from build123d import *

# Parameters (mm, degrees)
RESSALTO_EXTRUS_O1_DEPTH = 500
CANAL_DEPTH              = 800
ESBO_O2_5_R              = 2.1
FURO_DEPTH               = 501.49975025
CORTE_EXTRUS_O4_DEPTH    = 501.49975025
PADR_OCIRCULAR2_COUNT    = 3
PADR_OCIRCULAR2_ANGLE    = 180
ESPELHAR2_COPY_1_DEPTH   = 800
ESPELHAR2_COPY_2_DEPTH   = 800


with BuildPart() as part:
    # Esboço1 → Ressalto-extrusão1 (new body)
    with BuildSketch(Plane.XY):
        with BuildLine():
            Line((-19, 10), (19, 10))
            ThreePointArc((19, 10), (19.707106781, 9.707106781), (20, 9))
            Line((20, 9), (20, -9))
            ThreePointArc((20, -9), (19.707106781, -9.707106781), (19, -10))
            Line((19, -10), (-19, -10))
            ThreePointArc((-19, -10), (-19.707106781, -9.707106781), (-20, -9))
            Line((-20, -9), (-20, 9))
            ThreePointArc((-20, 9), (-19.707106781, 9.707106781), (-19, 10))
        make_face()
    extrude(amount=RESSALTO_EXTRUS_O1_DEPTH)

    # Esboço2 → CANAL (cut)
    with BuildSketch(Plane.XY.offset(500)):
        Polygon((-14.8, 10), (-13, 8.2), (-15.5, 8.2), (-15.5, 6.560660172), (-12.939339828, 4), (-10.3, 4), (-10, 3.7), (-9.7, 4), (-7.060660172, 4), (-4.5, 6.560660172), (-4.5, 8.2), (-7, 8.2), (-5.2, 10), align=None)
    canal = extrude(amount=-CANAL_DEPTH, mode=Mode.SUBTRACT)

    # Esboço2<5> → FURO (cut, through all)
    with BuildSketch(Plane.XY.offset(500)):
        with Locations((-10, 0)):
            Circle(ESBO_O2_5_R)
    furo = extrude(amount=-FURO_DEPTH, mode=Mode.SUBTRACT)

    # Esboço2<6> → Corte-extrusão4 (cut, through all)
    with BuildSketch(Plane.XY.offset(500)):
        Polygon((-2.7, 8.2), (-2.7, 6.239339828), (-6, 2.939339828), (-6, 0), (6, 0), (6, 2.939339828), (2.7, 6.239339828), (2.7, 8.2), align=None)
    corte_extrus_o4 = extrude(amount=-CORTE_EXTRUS_O4_DEPTH, mode=Mode.SUBTRACT)

    # PadrãoCircular2: CANAL ×3 about axis
    padr_ocircular2_axis = Axis((-10, 0, 0), (0, 0, 1))
    for i in range(1, PADR_OCIRCULAR2_COUNT):
        add(canal.rotate(padr_ocircular2_axis, i * PADR_OCIRCULAR2_ANGLE / (PADR_OCIRCULAR2_COUNT - 1)), mode=Mode.SUBTRACT)

    # Espelhar2: CANAL, FURO, Corte-extrusão4 across plane
    add(canal.mirror(Plane(origin=(0, 0, 0), x_dir=(0, 0, 1), z_dir=(1, 0, 0))), mode=Mode.SUBTRACT)
    add(furo.mirror(Plane(origin=(0, 0, 0), x_dir=(0, 0, 1), z_dir=(1, 0, 0))), mode=Mode.SUBTRACT)
    add(corte_extrus_o4.mirror(Plane(origin=(0, 0, 0), x_dir=(0, 0, 1), z_dir=(1, 0, 0))), mode=Mode.SUBTRACT)

    # Espelhar2 copy 1 sketch → Espelhar2 copy 1 (cut)
    with BuildSketch(Plane(origin=(10, 10, 500), x_dir=(0, 1, 0), z_dir=(0, 0, 1))):
        Polygon((-14.8, -10), (-13, -8.2), (-15.5, -8.2), (-15.5, -6.560660172), (-12.939339828, -4), (-10.3, -4), (-10, -3.7), (-9.7, -4), (-7.060660172, -4), (-4.5, -6.560660172), (-4.5, -8.2), (-7, -8.2), (-5.2, -10), align=None)
    extrude(amount=-ESPELHAR2_COPY_1_DEPTH, mode=Mode.SUBTRACT)

    # Espelhar2 copy 2 sketch → Espelhar2 copy 2 (cut)
    with BuildSketch(Plane(origin=(20, 0, 500), x_dir=(1, 0, 0), z_dir=(0, 0, 1))):
        Polygon((-14.8, -10), (-13, -8.2), (-15.5, -8.2), (-15.5, -6.560660172), (-12.939339828, -4), (-10.3, -4), (-10, -3.7), (-9.7, -4), (-7.060660172, -4), (-4.5, -6.560660172), (-4.5, -8.2), (-7, -8.2), (-5.2, -10), align=None)
    extrude(amount=-ESPELHAR2_COPY_2_DEPTH, mode=Mode.SUBTRACT)

    # Espelhar3: Corte-extrusão4 across plane
    add(corte_extrus_o4.mirror(Plane.ZX), mode=Mode.SUBTRACT)


solid = part.part
Design review of the part built by this model. Coordinates are the model's own, in mm. Coordinates: 2 decimals unless noted, no trailing zeros. One line per item, written item: value.
1) Mouldability with a two-part tool opening along Z and no side actions: class faces 1 (the face through (5, 5, 500)), 2 (the face through (5, 5, 0)), 3 (the face through (0, 10, 246)) as +Z half, -Z half, draft (parallel to the pull), parting line (faces both ways), or undercut.
Answer sheet:
face 1: +Z half
face 2: -Z half
face 3: draft
2) Add section A-A (z = 359.5). Give the number of separate pieces and of enclosed holes in the cut face, plus the area to 3 significant figures.
Answer sheet:
separate pieces: 1
enclosed holes: 3
area: 300 mm2
3) Insertion check: pin 1 (1.3 mm diameter, centred on x = 9, z = 242, fed in from -Y); pin 2 (3 mm diameter, centred on y = -0.5, z = 233, fed in from +X); pin 3 (0.8 mm diameter, centred on x = -14, z = 184, fed in from -Y). Each pin has a flat end and moves straight along its axis. Give the tip position at first contact, or say it passes through.
Answer sheet:
pin 1: stops at y = -4
pin 2: stops at x = 14
pin 3: stops at y = -9.6
4) To check wall thickness, follow probe 1 along Y at (x, z) = (15, 245); probe 2 along Y at (x, z) = (2, 467.5); probe 3 along Y at (x, z) = (10, 343). State the ranges of each line that lie inside material, in increasing order.
Answer sheet:
probe 1: y = -10 to -8.2, -6.06 to -3.94, 3.94 to 6.06, 8.2 to 10
probe 2: y = -10 to -8.2, 8.2 to 10
probe 3: y = -3.7 to -2.1, 2.1 to 3.7
